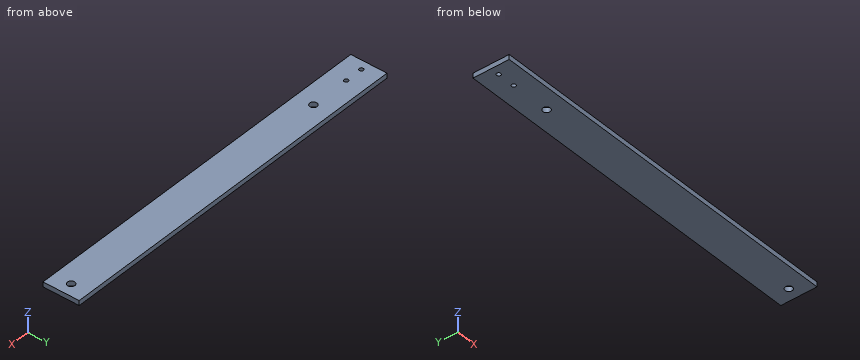
```python
from build123d import *

# Parameters (mm, degrees)
SKETCH_1_W             = 610
SKETCH_1_H             = 60
EXTRUDE_1_DEPTH        = 8
MM_1_D                 = 12
PATTERN_LINEAR_1_COUNT = 2
PATTERN_LINEAR_1_PITCH = 480
MM_2_D                 = 6.8
PATTERN_LINEAR_2_COUNT = 2
PATTERN_LINEAR_2_PITCH = 30


with BuildPart() as part:
    # 草图1 → 凸台-拉伸1 (new body)
    with BuildSketch(Plane.XY):
        Rectangle(SKETCH_1_W, SKETCH_1_H)
    extrude(amount=EXTRUDE_1_DEPTH)

    # 大小mm 暗销孔1 (through all)
    with Locations(Plane(origin=(285, 0, 8), x_dir=(1, 0, 0), z_dir=(0, 0, 1))):
        with Locations((0, 0)):
            mm_1 = Hole(MM_1_D / 2)

    # 阵列(线性)1: 大小mm 暗销孔1 ×2
    with Locations(*[(-i * PATTERN_LINEAR_1_PITCH, 0, 0) for i in range(1, PATTERN_LINEAR_1_COUNT)]):
        add(mm_1, mode=Mode.SUBTRACT)

    # 大小mm 暗销孔2 (through all)
    with Locations(Plane(origin=(-290, 0, 8), x_dir=(1, 0, 0), z_dir=(0, 0, 1))):
        with Locations((0, 0)):
            mm_2 = Hole(MM_2_D / 2)

    # 阵列(线性)2: 大小mm 暗销孔2 ×2
    with Locations(*[(i * PATTERN_LINEAR_2_PITCH, 0, 0) for i in range(1, PATTERN_LINEAR_2_COUNT)]):
        add(mm_2, mode=Mode.SUBTRACT)


solid = part.part
```
Read the model definition and answer for the solid it produces. Units are mm, in the model's axes. Give positions to 0.01 mm unless a question says otherwise; leave off trailing zeros. Loops run counter-clockwise (first coordinate to the right, second up) from the corner with the lowest first, then second, coordinate; pieces in that order, holes last.
Item 1: The part is cut by section A-A (x = 285). Write down the section's boundary in (y, z), and give its area (3 significant figures).
Item 2: This flat-tipped pin is pushed along its axis until it touches: pin 1 Ø9.5 at (x, y) = (285, 0) entering from -Z. Where does it stop, or does it pass through?
Item 3: Find the intervals of material crossed by line 1 along Y through (x, z) = (-195, 4); line 2 along Y through (x, z) = (-260, 2.75); line 3 along X through (y, z) = (-1.5, 2.5), in increasing order.
Taken from the geometry:
1. outline: (-30, 0) - (-6, 0) - (-6, 8) - (-30, 8) - close; (6, 0) - (30, 0) - (30, 8) - (6, 8) - close
1. area: 384 mm2
2. pin 1: passes through
3. line 1: y = -30 to -6, 6 to 30
3. line 2: y = -30 to -3.4, 3.4 to 30
3. line 3: x = -305 to -293.05, -286.95 to -263.05, -256.95 to -200.81, -189.19 to 279.19, 290.81 to 305
